```python
from build123d import *

# Parameters (mm, degrees)
SKETCH1_R           = 31
BOSS_EXTRUDE1_DEPTH = 110
SHELL1_T            = -1
FILLET2_R           = 5


with BuildPart() as part:
    # Sketch1 → Boss-Extrude1 (new body)
    with BuildSketch(Plane.XY):
        with Locations((-27.512537488, 7.30607002)):
            Circle(SKETCH1_R)
    extrude(amount=BOSS_EXTRUDE1_DEPTH)

    # Shell1
    shell1_openings = [part.faces().sort_by_distance(p)[0] for p in [
        (3.487462512, 7.30607002, 110),
    ]]
    offset(amount=SHELL1_T, openings=shell1_openings, kind=Kind.INTERSECTION)

    # Fillet2
    fillet2_edges = [part.edges().sort_by_distance(p)[0] for p in [
        (-58.512537488, 7.30607002, 0),
    ]]
    fillet(fillet2_edges, radius=FILLET2_R)


solid = part.part
```
Geometry: final body of the model. Coordinates: model frame, mm. Coordinates: 2 decimals unless noted, no trailing zeros. Order: outer loops, then holes, each group sorted by start corner. A loop starts at its lowest first (then second) coordinate and runs counter-clockwise, first axis right, second up. Notation, with made-up numbers: M 31.25,54.5 L 53.25,54.5 A21 cw 53.25,66.5 Z; hole C -1,19.25 d10. An arc over 180 degrees is marked long. Answer in a Markdown table with one row per item. Add a question column.
Q1. Section query C-C on z = 89.5. Return the cut outline in (x, y), and give its area (3 significant figures).
Q2. Line query: L1, parallel to Z at x = -18, y = -15.5; L2, parallel to X at y = 1.5, z = 55.5; L3, parallel to X at y = 7, z = 104.5. Output: solid intervals per line, ascending.
Q3. Contact query for flat-ended pins moving along their axis: P1, Ø12, axis at y = -5.5, z = 21.5, coming from the -X side; P2, Ø6, axis at x = -36, z = 35.5, coming from the -Y side; P3, Ø1.5, axis at y = -7, z = 97.5, coming from the +X side. Output: stop coordinate, or through.
Q4. Mould query, pull axis X, two halves, no side actions, for faces 1 (the cylindrical face through (2.056, 16.618, 56.765)), 2 (the cylindrical face through (0.2, -4.18, 54.74)), 3 (the flat face through (-28, 8, 1)), 4 (the flat face through (-44, 33, 110)). Classes: released by +X, released by -X, zero draft, split by the parting line, or undercut.
Completed:
| question | item | result |
|---|---|---|
| 1 | outline | C -27.51,7.31 d62; hole C -27.51,7.31 d60 |
| 1 | area | 192 mm2 |
| 2 | L1 | z = 0 to 1 |
| 2 | L2 | x = -57.96 to -56.95, 1.92 to 2.94 |
| 2 | L3 | x = -58.51 to -57.51, 2.49 to 3.49 |
| 3 | P1 | stops at x = -57.76 |
| 3 | P2 | stops at y = -23.2 |
| 3 | P3 | stops at x = 0.37 |
| 4 | face 1 | split by the parting line |
| 4 | face 2 | undercut |
| 4 | face 3 | undercut |
| 4 | face 4 | zero draft |
